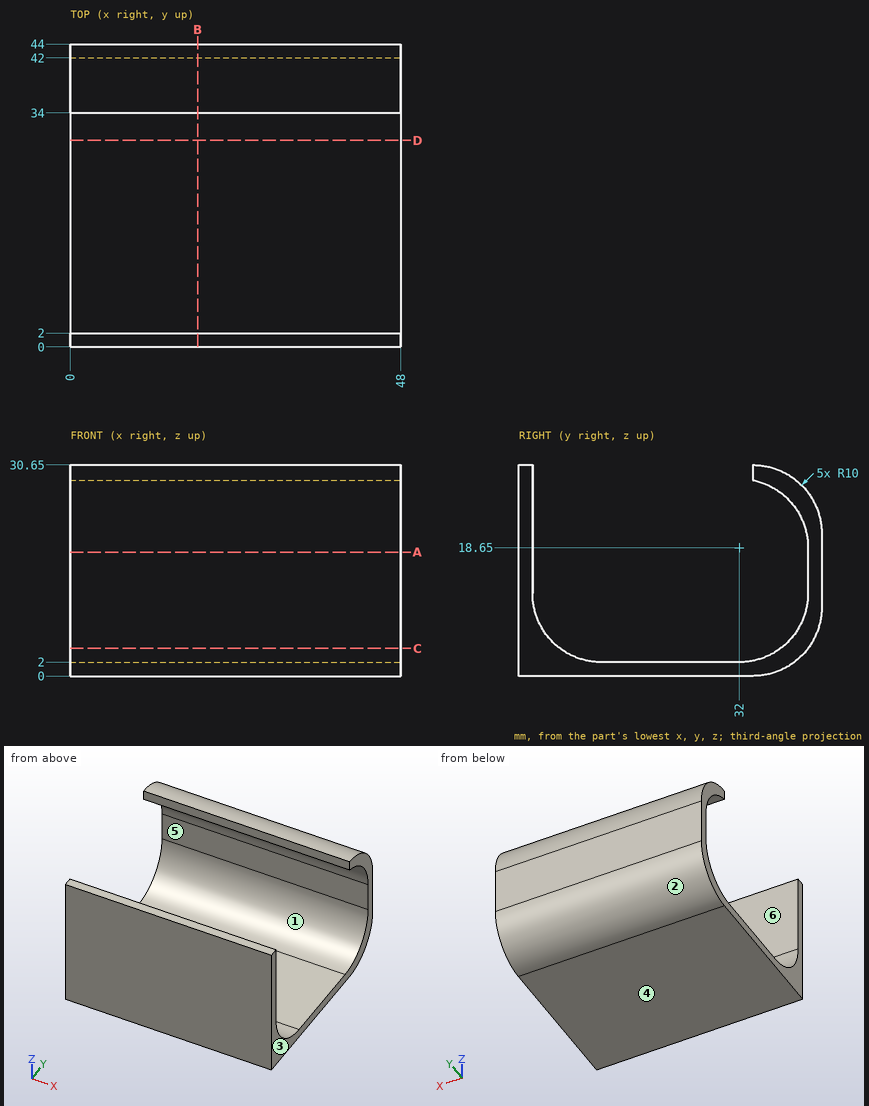
Input: dimensioned drawing with shaded views. Units: mm. Origin: part minimum x, y, z. A direction names the side the tool comes from. Give positions to 0.01 mm unless a question says otherwise; leave off trailing zeros. Loops run counter-clockwise (first coordinate to the right, second up) from the corner with the lowest first, then second, coordinate; pieces in that order, holes last. Notation, with made-up numbers: (80.25, 15) -> (133.25, 15) arc R24 ccw to (133.25, 28) -> close; hole circle Ø2 at (86.5, 78). An arc over 180 degrees is marked (long way). Use a Markdown table: item, result. Add a question column.
1) Section query A-A, the plane z = 18. Return the cut outline in (x, y), then the cut area to 3 significant figures.
2) Reachability of the marked faces 4, 5 and 6 from +Z, -Z, +X, -X, +Y, -Y: full face, straight path, thin tool, end or side. Return the list, or none.
3) First-contact query: pin 1 (6 mm diameter, centred on x = 28, y = 22.5, fed in from +Z); pin 2 (1.5 mm diameter, centred on x = 27, z = 7, fed in from +Y). Flat tips, straight axial feed; report the tip coordinate or a pass-through.
4) Pull-direction query (Z, two-part tool) for the marked faces 1, 2 and 3; classes: +Z half, -Z half, draft (parallel to the pull), parting line (faces both ways), or undercut.
5) Section query C-C, the plane z = 4. Return the cut outline in (x, y), then the cut area to 3 significant figures.
6) Line query: line 1 along Y through (x, z) = (6.5, 17); line 2 along Z through (x, y) = (33, 21); line 3 along Y through (x, z) = (44, 24.5). Output: solid intervals per line, ascending. Write a range as [from, to].
7) Section query B-B, the plane x = 18.5. Return the cut outline in (y, z), then the cut area to 3 significant figures.
8) Section query D-D, the plane y = 30. Return the cut outline in (x, z).
Numbers:
| question | item | result |
|---|---|---|
| 1 | outline | (0, 0) -> (48, 0) -> (48, 2) -> (0, 2) -> close; (0, 42) -> (48, 42) -> (48, 44) -> (0, 44) -> close |
| 1 | area | 192 mm2 |
| 2 | face 4 | -Z, +X, -X, +Y, -Y |
| 2 | face 5 | +X, -X |
| 2 | face 6 | +Z, +X, -X |
| 3 | pin 1 | stops at z = 2 |
| 3 | pin 2 | stops at y = 43.74 |
| 4 | face 1 | undercut |
| 4 | face 2 | -Z half |
| 4 | face 3 | draft |
| 5 | outline | (0, 0) -> (48, 0) -> (48, 6) -> (0, 6) -> close; (0, 38) -> (48, 38) -> (48, 42) -> (0, 42) -> close |
| 5 | area | 480 mm2 |
| 6 | line 1 | y = [0, 2], [42, 44] |
| 6 | line 2 | z = [0, 2] |
| 6 | line 3 | y = [0, 2], [40.11, 43.23] |
| 7 | outline | (0, 0) -> (34, 0) arc R10 ccw to (44, 10) -> (44, 20.65) arc R10 ccw to (34, 30.65) -> (34, 28.45) arc R10 cw to (42, 18.65) -> (42, 12) arc R10 cw to (32, 2) -> (12, 2) arc R10 cw to (2, 12) -> (2, 30.65) -> (0, 30.65) -> close |
| 7 | area | 240 mm2 |
| 8 | outline | (0, 0) -> (48, 0) -> (48, 2) -> (0, 2) -> close |
